Build history of the part. All positions in model axes, mm. A direction names the side the tool comes from. Round coordinates to 2 decimals unless told otherwise and drop trailing zeros. Loops run counter-clockwise (first coordinate to the right, second up) from the corner with the lowest first, then second, coordinate; pieces in that order, holes last.
from build123d import *

# Parameters (mm, degrees)
ESQUISSE1_W   = 20
ESQUISSE1_H   = 10
ESQUISSE1_W_2 = 18
ESQUISSE1_H_2 = 8


with BuildPart() as part:
    # Balayage1: sweep along a path in Esquisse2
    with BuildLine(Plane(origin=(0, 0, 0), x_dir=(0, 0, -1), z_dir=(1, 0, 0))) as balayage1_path:
        Line((0, 2.284569244), (250, 2.284569244))
        ThreePointArc((250, 2.284569244), (278, 30.284569244), (250, 58.284569244))
        Line((250, 58.284569244), (220, 58.284569244))
    # Esquisse1 → Balayage1 (sweep)
    with BuildSketch(Plane.XY):
        with Locations((10, 5)):
            Rectangle(ESQUISSE1_W, ESQUISSE1_H)
        with Locations((10, 5)):
            Rectangle(ESQUISSE1_W_2, ESQUISSE1_H_2, mode=Mode.SUBTRACT)
    sweep(path=balayage1_path.line)


solid = part.part
(1) Pull direction Z, two halves, no side cores. Call faces 5 (the face through (9.86, 29.84, -270.28)), 6 (the face through (10.13, 29.82, -271.28)), 7 (the face through (10.14, 29.619, -280.277)), 8 (the face through (0, 8, -172)): +Z half, -Z half, draft (parallel to the pull), parting line (faces both ways), or undercut.
Responses:
face 5: +Z half
face 6: undercut
face 7: -Z half
face 8: draft
(2) Slice it at D-D on z = -153. List the corners of the cut face in (x, y).
Responses:
outline: (0, 0) - (20, 0) - (20, 10) - (0, 10) - close; hole (1, 1) - (19, 1) - (19, 9) - (1, 9) - close
(3) Probe line 1 (X direction, y = 7.5, z = -260); line 2 (Y direction, x = 15.75, z = -71.5); line 3 (Y direction, x = 1.5, z = -230.5). List the from-to ranges inside material, lowest first.
Responses:
line 1: x = 0 to 1, 19 to 20
line 2: y = 0 to 1, 9 to 10
line 3: y = 0 to 1, 9 to 10, 50.57 to 51.57, 59.57 to 60.57
(4) Slice it at C-C on y = 42.5. List the corners of the cut face in (x, z).
Responses:
outline: (0, -277.71) - (20, -277.71) - (20, -266.19) - (0, -266.19) - close; hole (1, -276.62) - (19, -276.62) - (19, -267.43) - (1, -267.43) - close
(5) Slice it at A-A on z = -239. List the corners of the cut face in (x, y), plus the area to 3 significant figures.
Responses:
outline: (0, 0) - (20, 0) - (20, 10) - (0, 10) - close; (0, 50.57) - (20, 50.57) - (20, 60.57) - (0, 60.57) - close; hole (1, 1) - (19, 1) - (19, 9) - (1, 9) - close; hole (1, 51.57) - (19, 51.57) - (19, 59.57) - (1, 59.57) - close
area: 112 mm2
(6) Slice it at B-B on x = 7.5. List the corners of the cut face in (y, z).
Responses:
outline: (0, -250) arc R30.28 ccw to (60.57, -250) - (60.57, -220) - (59.57, -220) - (59.57, -250) arc R29.28 cw to (1, -250) - (1, 0) - (0, 0) - close; (9, -250) arc R21.28 ccw to (51.57, -250) - (51.57, -220) - (50.57, -220) - (50.57, -250) arc R20.28 cw to (10, -250) - (10, 0) - (9, 0) - close
(7) Which spindle directions (+Z, -Z, +X, -X, +Y, -Y) get a long thin tool onto all of the face, cutting with end or side? Do faces 1 (the face through (10, 50.569, -235)), 2 (the face through (10, 60, -220)), 3 (the face through (9.874, 29.641, -279.277)), 4 (the face through (10, 1, -127)). Say none if no direction does.
Responses:
face 1: +Z, +X, -X
face 2: +Z, +X, -X, +Y
face 3: none
face 4: +Z
(8) Pin check, flat tips, straight feed: P1, Ø5.5, axis at x = 12, z = -98.5, coming from the +Y side; P2, Ø10, axis at x = 3, y = 21.5, coming from the -Z side; P3, Ø6, axis at x = 10, y = 35.5, coming from the +Z side. Stop position of each tip, or through.
Responses:
P1: stops at y = 10
P2: stops at z = -280.05
P3: stops at z = -268.55
